Check sheet for the modelled part. Datum: model origin and axes. Units: mm. Give positions to 0.01 mm unless a question says otherwise; leave off trailing zeros. Write each loop counter-clockwise with the first axis right and the second up, starting at its lowest first coordinate (ties: lowest second). Pieces come first, ordered by that corner, then holes. Notation, with made-up numbers: (-15.75, -23.5) -> (2.25, -23.5) arc R25 ccw to (2.25, 0.5) -> close; hole circle Ø3 at (74.5, 33.5). An arc over 180 degrees is marked (long way). Use a Markdown table: item, result. Add a question column.
1. Gauge pin test, flat end, axial feed: P1, Ø10, axis at x = -20.066, z = -19.05, coming from the -Y side. Record the tip position at first contact, or that the pin passes through.
2. Release check for a two-part mould opening along Z. For faces 1 (the cylindrical face through (30.539, 2.755, -16.233)), 2 (the cylindrical face through (32.69, 2.75, -54.05)), 3 (the flat face through (-2, 3, 114.3)), 4 (the cylindrical face through (-112.49, 2.83, -112.39)) record: released by +Z, released by -Z, zero draft, split by the parting line, or undercut.
3. Scan line: probe 1 along Z at (x, y) = (31.5, 1.55). Record every from-to range of solid material in increasing order. Write a range as [from, to].
4. Cross-section at A-A (z = 19.05). Enter the section's corners in (x, y), then the cut area to 3 significant figures.
from build123d import *

# Parameters (mm, degrees)
SKETCH1_W                   = 228.6
SKETCH1_H                   = 228.6
BOSS_EXTRUDE1_DEPTH         = 5.588
F_1_4_0_25_DIAMETER_HOLE1_D = 6.35
LPATTERN1_COUNT             = 4
LPATTERN1_PITCH             = 38.1
FILLET1_R                   = 6.35


with BuildPart() as part:
    # Sketch1 → Boss-Extrude1 (new body)
    with BuildSketch(Plane(origin=(0, 0, 0), x_dir=(1, 0, 0), z_dir=(0, 1, 0))):
        Rectangle(SKETCH1_W, SKETCH1_H)
    extrude(amount=BOSS_EXTRUDE1_DEPTH)

    # 1/4 (0.25) Diameter Hole1 (through all)
    with Locations(Plane(origin=(0, 5.588, 0), x_dir=(1, 0, 0), z_dir=(0, 1, 0))):
        with Locations((-20.066, 57.15), (32.004, 57.15)):
            f_1_4_0_25_diameter_hole1 = Hole(F_1_4_0_25_DIAMETER_HOLE1_D / 2)

    # LPattern1: 1/4 (0.25) Diameter Hole1 ×4
    with Locations(*[(0, 0, i * LPATTERN1_PITCH) for i in range(1, LPATTERN1_COUNT)]):
        add(f_1_4_0_25_diameter_hole1, mode=Mode.SUBTRACT)

    # Fillet1
    fillet1_edges = [part.edges().sort_by_distance(p)[0] for p in [
        (-114.3, 2.794, -114.3),
        (114.3, 2.794, -114.3),
        (114.3, 2.794, 114.3),
        (-114.3, 2.794, 114.3),
    ]]
    fillet(fillet1_edges, radius=FILLET1_R)


solid = part.part
Worked answers:
| question | item | result |
|---|---|---|
| 1 | P1 | stops at y = 0 |
| 2 | face 1 | undercut |
| 2 | face 2 | undercut |
| 2 | face 3 | released by +Z |
| 2 | face 4 | released by -Z |
| 3 | probe 1 | z = [-114.3, -60.28], [-54.02, -22.18], [-15.92, 15.92], [22.18, 54.02], [60.28, 114.3] |
| 4 | outline | (-114.3, 0) -> (-23.24, 0) -> (-23.24, 5.59) -> (-114.3, 5.59) -> close; (-16.89, 0) -> (28.83, 0) -> (28.83, 5.59) -> (-16.89, 5.59) -> close; (35.18, 0) -> (114.3, 0) -> (114.3, 5.59) -> (35.18, 5.59) -> close |
| 4 | area | 1,210 mm² |
